Autodesk Fusion 360 part; units mm, degrees
sketch "Sketch4" plane through (0, 0, 0) normal (0, 0, 1) x (1, 0, 0)
  line L0 (-200, 100) -> (-175, 100)
  line L1 (-175, 100) -> (-175, -60)
  line L2 (-175, -60) -> (-200, -60)
  line L3 (-200, -60) -> (-200, 100)
  dimension "d3" = 25
  dimension "d4" = 160
extrude "Extrude1" add sketch "Sketch4" along normal blind 20
sketch "Sketch5" plane through (0, 0, 20) normal (0, 0, 1) x (-1, 0, 0)
  line L0 (200, 60) -> (175, 60)
  line L1 (175, 60) -> (175, -100)
  line L2 (175, -100) -> (200, -100)
  line L3 (200, -100) -> (200, 60)
  circle A0 centre (187.5, -80) radius 8.0085
  dimension "d8" = 16.017
extrude "Extrude2" cut sketch "Sketch5" against normal blind 55 contours A0
fillet "Fillet1" radius 7 2 edges at (-187.5, 100, 20) (-187.5, 100, 0)
sketch "Sketch11" plane through (0, 0, 20) normal (0, 0, 1) x (-1, 0, 0)
  line L0 (200, -93) -> (200, 60)
  line L1 (200, 60) -> (175, 60)
  line L2 (175, 60) -> (175, -93)
  circle A0 centre (187.5, -80) radius 8.0085
  line L3 (187.5, -80) -> (179.4991, -88.0009)
  line L4 (187.5, -80) -> (195.5009, -88.0009)
  line L5 (187.5, -80) -> (195.5009, -71.9991)
  line L6 (187.5, -80) -> (179.4991, -71.9991)
  line L7 (175, -93) -> (200, -93)
hole "Hole2" at (-179.4991, 71.9991, 20) at (-179.4991, 88.0009, 20) at (-195.5009, 88.0009, 20) at (-195.5009, 71.9991, 20) direction (0, 0, -1) diameter 1.623 depth 20 tip angle 180 counterbore diameter 3.9 counterbore depth 1
sketch "Sketch13" plane through (0, -60, 0) normal (0, -1, 0) x (1, 0, 0)
  line L0 (-200, 0) -> (-175, 0)
  line L1 (-175, 0) -> (-175, 20)
  line L2 (-175, 20) -> (-200, 20)
  line L3 (-200, 20) -> (-200, 0)
  circle A0 centre (-187.5, 10) radius 8
  dimension "d46" = 16
extrude "Extrude8" add sketch "Sketch13" along normal blind 25 contours A0
sketch "Sketch14" plane through (0, -85, 0) normal (0, -1, 0) x (1, 0, 0)
  circle A0 centre (-187.5, 10) radius 8
  circle A1 centre (-187.5, 10) radius 2.0005
  dimension "d49" = 4.001
extrude "Extrude9" cut sketch "Sketch14" against normal blind 15 contours A1
sketch "Sketch16" plane through (0, -85, 0) normal (0, -1, 0) x (1, 0, 0)
  circle A0 centre (-187.5, 10) radius 2.0005
  circle A1 centre (-187.5, 10) radius 8
  curve A2
hole "Hole4" at (-187.5, -75.0094, 18) direction (0, 0, -1) diameter 1.623 end through all counterbore diameter 4 counterbore depth 1
component "4124A15_7-1 4 Diameter Smooth-Cut Circular Saw Blade for Wood" placed x (1, 0, 0) y (0, 1, 0) z (0, 0, 1) at (0, 0, 0)
component "6343K96_Bearing Locknut" placed x (1, 0, 0) y (0, 0, -1) z (0, 1, 0) at (-164.7507, -187.0518, -22.2618)
component "6627T34_Stepper Motor" placed x (1, 0, 0) y (0, 1, 0) z (0, 0, 1) at (-161.9415, -183.813, -21.8716)
The model under review builds one solid part; all positions refer to its coordinate system, in mm. A direction names the side the tool comes from. Coordinates: 2 decimals unless noted, no trailing zeros. Write each loop counter-clockwise with the first axis right and the second up, starting at its lowest first coordinate (ties: lowest second). Pieces come first, ordered by that corner, then holes. Notation, with made-up numbers: (-5, -5.5) - (31, -5.5) arc R29 cw to (31, 20.5) - close; hole circle Ø5 at (71, 60.25). An arc over 180 degrees is marked (long way). Answer as a JSON object with one key per item and string values. Group by question number.
1. Mouldability with a two-part tool opening along Z and no side actions: class faces 1 (the face through (-187.934, -77.605, 8.047)), 2 (the face through (-188, -70, 10)), 3 (the face through (-193.77, 71.1, 19.49)), 4 (the face through (-187.3, 97.9, 2)) as pulls with the +Z half, pulls with the -Z half, needs draft (parallel to the pull), parting line crosses it, or undercut.
2. To check wall thickness, follow probe 1 along Y at (x, z) = (-194.5, 19.25); probe 2 along Y at (x, z) = (-187.5, 5.5); probe 3 along Y at (x, z) = (-179, 10.75). State the ranges of each line that lie inside material, in increasing order.
3. Clearance check with flat-ended pins moving along their axes: pin 1 Ø4.5 at (x, y) = (-187, -75.5) entering from +Z; pin 2 Ø1 at (x, z) = (-195, 15) entering from -Y; pin 3 Ø1.2 at (x, z) = (-187, 9.5) entering from -Y. State where each tip first meets the part, or that it passes through.
4. Add section A-A (y = 80). Give the boundary of the cut face in (x, z).
5. Machinability: for faces 5 (the face through (-177.77, 71.1, 19.49)), 6 (the face through (-188, 100, 10)), 7 (the face through (-196, -60, 10)), which of the approach directions +Z, -Z, +X, -X, +Y, -Y give a long, thin tool a straight path to every point of the face, cutting with its end or side? Answer none if there is none.
6. Add section B-B (z = 10). Give the boundary of the cut face in (x, y).
Findings:
{
 "1": {"face 1": "undercut", "face 2": "undercut", "face 3": "needs draft", "face 4": "pulls with the -Z half"},
 "2": {"probe 1": "-60 to 70.33, 73.67 to 76.11, 83.89 to 86.33, 89.67 to 96.15", "probe 2": "-85 to -75.82, -74.2 to 71.99, 88.01 to 99.84", "probe 3": "-60 to 71.36, 72.64 to 87.36, 88.64 to 100"},
 "3": {"pin 1": "z = 18", "pin 2": "y = -60", "pin 3": "y = -70"},
 "4": {"outline": "(-200, 0) - (-195.51, 0) - (-195.51, 20) - (-200, 20) - close; (-179.49, 0) - (-175, 0) - (-175, 20) - (-179.49, 20) - close"},
 "5": {"face 5": "+Z", "face 6": "+Z, -Z, +X, -X, +Y", "face 7": "-Y"},
 "6": {"outline": "(-200, -60) - (-195.5, -60) - (-195.5, -85) - (-189.5, -85) - (-189.5, -70) - (-185.5, -70) - (-185.5, -85) - (-179.5, -85) - (-179.5, -60) - (-175, -60) - (-175, 100) - (-200, 100) - close; hole circle Ø1.62 at (-195.5, 72); hole circle Ø1.62 at (-195.5, 88); hole circle Ø16.02 at (-187.5, 80); hole circle Ø1.62 at (-179.5, 72); hole circle Ø1.62 at (-179.5, 88)"}
}
